Verification items for the finished model (mm, model axes). Face numbers are marked on the shaded views. Give positions to 0.01 mm unless a question says otherwise; leave off trailing zeros. Loops run counter-clockwise (first coordinate to the right, second up) from the corner with the lowest first, then second, coordinate; pieces in that order, holes last. Notation, with made-up numbers: (18, 49) -> (35, 49) arc R23 ccw to (35, 66) -> close; hole circle Ø2 at (68.25, 7). An arc over 180 degrees is marked (long way). Answer in a Markdown table with one row per item. Add a question column.
Q1. Section check C-C on z = -14. Enter the section's corners in (x, y).
Q2. Gauge pin test, flat ends, axial feed: P1, Ø3, axis at x = 2.5, z = -12, coming from the +Y side; P2, Ø7.5, axis at x = 10, y = 7.5, coming from the +Z side; P3, Ø7.5, axis at x = -2.5, z = 0, coming from the +Y side. Record the tip position at first contact, or that the pin passes through.
Q3. Section check B-B on z = 7.5. Enter the section's corners in (x, y), and give its area (3 significant figures).
Q4. Section check D-D on x = 18.5. Enter the section's corners in (y, z), and give its area (3 significant figures).
Q5. Release check for a two-part mould opening along Y. For the marked faces 1, 2, 3 and 4 record: pulls with the +Y half, pulls with the -Y half, needs draft (parallel to the pull), parting line crosses it, or undercut.
Q6. Section check A-A on x = 0. Enter the section's corners in (y, z), and give its area (3 significant figures).
Q7. Material ranges on probe 1 along X at (y, z) = (15, -13.7); probe 2 along Z at (x, y) = (4, 22); probe 3 along Z at (x, y) = (-18.5, -1.2), recorded low to high.
```python
from build123d import *

# Parameters (mm, degrees)
F0_W     = 47
F0_H     = 25
F0_R     = 1.5
F1_DEPTH = 5
F2_R     = 2.5
F2_W     = 47
F2_H     = 5
F3_DEPTH = 5


with BuildPart() as f1:
    # F0 (on Front) → F1 (new body)
    with BuildSketch(Plane.XZ):
        Rectangle(F0_W, F0_H)
        with Locations((-18.5, -7.5)):
            Circle(F0_R, mode=Mode.SUBTRACT)
        with Locations((18.5, 7.5)):
            Circle(F0_R, mode=Mode.SUBTRACT)
    extrude(amount=F1_DEPTH)

    # F2 (on face) → F3 (join)
    with BuildSketch(Plane(origin=(0, 0, -12.5), x_dir=(1, 0, 0), z_dir=(0, 0, -1))):
        with BuildLine():
            Line((23.5, 0), (-23.5, 0))
            Line((-23.5, 0), (-23.5, -15))
            ThreePointArc((-23.5, -15), (-20.571068, -22.071068), (-13.5, -25))
            Line((-13.5, -25), (13.5, -25))
            ThreePointArc((13.5, -25), (20.571068, -22.071068), (23.5, -15))
            Line((23.5, -15), (23.5, 0))
        make_face()
        with Locations((0, -15)):
            Circle(F2_R, mode=Mode.SUBTRACT)
        with Locations((0, 2.5)):
            Rectangle(F2_W, F2_H)
    extrude(amount=F3_DEPTH)


solid = f1.part
```
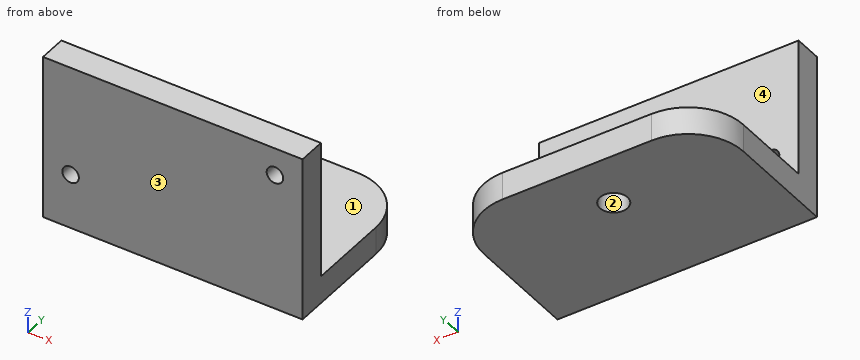
Taken from the geometry:
| question | item | result |
|---|---|---|
| 1 | outline | (-23.5, -5) -> (23.5, -5) -> (23.5, 15) arc R10 ccw to (13.5, 25) -> (-13.5, 25) arc R10 ccw to (-23.5, 15) -> close; hole circle Ø5 at (0, 15) |
| 2 | P1 | stops at y = 25 |
| 2 | P2 | stops at z = -12.5 |
| 2 | P3 | stops at y = 0 |
| 3 | outline | (-23.5, -5) -> (17, -5) -> (17, 0) -> (-23.5, 0) -> close; (20, -5) -> (23.5, -5) -> (23.5, 0) -> (20, 0) -> close |
| 3 | area | 220 mm² |
| 4 | outline | (-5, -17.5) -> (23.66, -17.5) -> (23.66, -12.5) -> (0, -12.5) -> (0, 6) -> (-5, 6) -> close; (-5, 9) -> (0, 9) -> (0, 12.5) -> (-5, 12.5) -> close |
| 4 | area | 253 mm² |
| 5 | face 1 | needs draft |
| 5 | face 2 | undercut |
| 5 | face 3 | pulls with the -Y half |
| 5 | face 4 | pulls with the +Y half |
| 6 | outline | (-5, -17.5) -> (12.5, -17.5) -> (12.5, -12.5) -> (0, -12.5) -> (0, 12.5) -> (-5, 12.5) -> close; (17.5, -17.5) -> (25, -17.5) -> (25, -12.5) -> (17.5, -12.5) -> close |
| 6 | area | 250 mm² |
| 7 | probe 1 | x = -23.5 to -2.5, 2.5 to 23.5 |
| 7 | probe 2 | z = -17.5 to -12.5 |
| 7 | probe 3 | z = -17.5 to -9, -6 to 12.5 |
